Work out the finished part from the listing and answer in its coordinate system (mm). A direction names the side the tool comes from. Coordinates: 2 decimals unless noted, no trailing zeros. Write each loop counter-clockwise with the first axis right and the second up, starting at its lowest first coordinate (ties: lowest second). Pieces come first, ordered by that corner, then holes. Notation, with made-up numbers: (65, 47.25) -> (71, 47.25) arc R31 cw to (71, 80.25) -> close; hole circle Ø3 at (-18, 12.5). An arc over 180 degrees is marked (long way). Write each question's results on one line, items separated by ' | '. Start each with the question number.
from build123d import *


with BuildPart() as part:
    # Sweep1: sweep along a path in Sketch1
    with BuildLine(Plane(origin=(0, 0, 0), x_dir=(1, 0, 0), z_dir=(0, 1, 0))) as sweep1_path:
        Line((279.4, -279.4), (-279.4, -279.4))
        Line((-279.4, -279.4), (-279.4, 279.4))
        Line((-279.4, 279.4), (279.4, 279.4))
        Line((279.4, 279.4), (279.4, -279.4))
    # Sketch2 → Sweep1 (sweep)
    with BuildSketch(Plane.XY):
        Polygon((-279.4, 0), (-241.3, 0), (-241.3, -38.1), (-247.65, -38.1), (-247.65, -6.35), (-279.4, -6.35), align=None)
    sweep(path=sweep1_path.line, transition=Transition.RIGHT)


solid = part.part
1. For faces 1 (the face through (-4, 0, -252)), 2 (the face through (247.65, -22, 3)), 3 (the face through (241.3, -19, 3)), 4 (the face through (-247.65, -22, -3)), determine the directions among +Z, -Z, +X, -X, +Y, -Y from which every point of the face is accessible in a straight line to the end or side of a thin tool.
2. Determine the mould class of faces 5 (the face through (3, -22, -247.65)), 6 (the face through (-3, -19, 241.3)), 7 (the face through (-3, -22, 247.65)), 8 (the face through (3, -19, -241.3)) for opening direction Z: pulls with the +Z half, pulls with the -Z half, needs draft (parallel to the pull), parting line crosses it, or undercut.
3. Find the intervals of material crossed by L1, parallel to X at y = -1.5, z = 203.5; L2, parallel to Z at x = 155, y = -6.5, in increasing order.
4. Given pin 1 Ø5 at (y, z) = (-19, -90.5) entering from +X; pin 2 Ø11.5 at (y, z) = (-22.5, 29) entering from +X; pin 3 Ø9.5 at (y, z) = (-20, 19) entering from -X, each flat-ended and moving along its own axis, determine where each tip first touches the part or whether it passes through.
5. Find section A-A on z = -180.5. Give the vertices of the cut face in (x, y).
6. Find section B-B on y = -25. Give the vertices of the cut face in (x, z).
7. Find section C-C on x = 123.5. Give the vertices of the cut face in (y, z), and give its area (3 significant figures).
Ans:
1) face 1: +Z, -Z, +X, -X, +Y | face 2: +Z, -Z, +X, -Y | face 3: +Y, -Y | face 4: +Z, -Z, -X, -Y
2) face 5: pulls with the -Z half | face 6: undercut | face 7: pulls with the +Z half | face 8: undercut
3) L1: x = -279.4 to -241.3, 241.3 to 279.4 | L2: z = -247.65 to -241.3, 241.3 to 247.65
4) pin 1: stops at x = 247.65 | pin 2: stops at x = 247.65 | pin 3: stops at x = -247.65
5) outline: (-279.4, -6.35) -> (-247.65, -6.35) -> (-247.65, -38.1) -> (-241.3, -38.1) -> (-241.3, 0) -> (-279.4, 0) -> close; (241.3, -38.1) -> (247.65, -38.1) -> (247.65, -6.35) -> (279.4, -6.35) -> (279.4, 0) -> (241.3, 0) -> close
6) outline: (-247.65, -247.65) -> (247.65, -247.65) -> (247.65, 247.65) -> (-247.65, 247.65) -> close; hole (-241.3, -241.3) -> (241.3, -241.3) -> (241.3, 241.3) -> (-241.3, 241.3) -> close
7) outline: (-38.1, -247.65) -> (-6.35, -247.65) -> (-6.35, -279.4) -> (0, -279.4) -> (0, -241.3) -> (-38.1, -241.3) -> close; (-38.1, 241.3) -> (0, 241.3) -> (0, 279.4) -> (-6.35, 279.4) -> (-6.35, 247.65) -> (-38.1, 247.65) -> close | area: 887 mm²
